```python
from build123d import *

# Parameters (mm, degrees)
SKETCH1_R           = 7.9375
SKETCH1_R_2         = 4.9657
BOSS_EXTRUDE1_DEPTH = 0.8128
FILLET1_R           = 0.32512


with BuildPart() as part:
    # Sketch1 → Boss-Extrude1 (new, symmetric)
    with BuildSketch(Plane(origin=(0, 0, 0), x_dir=(0, 0, -1), z_dir=(1, 0, 0))):
        Circle(SKETCH1_R)
        Circle(SKETCH1_R_2, mode=Mode.SUBTRACT)
    extrude(amount=BOSS_EXTRUDE1_DEPTH, both=True)

    # Fillet1
    fillet1_edges = [part.edges().sort_by_distance(p)[0] for p in [
        (-0.8128, 0, 7.9375),
        (0.8128, 0, 7.9375),
        (-0.8128, 0, 4.9657),
        (0.8128, 0, 4.9657),
    ]]
    fillet(fillet1_edges, radius=FILLET1_R)


solid = part.part
```
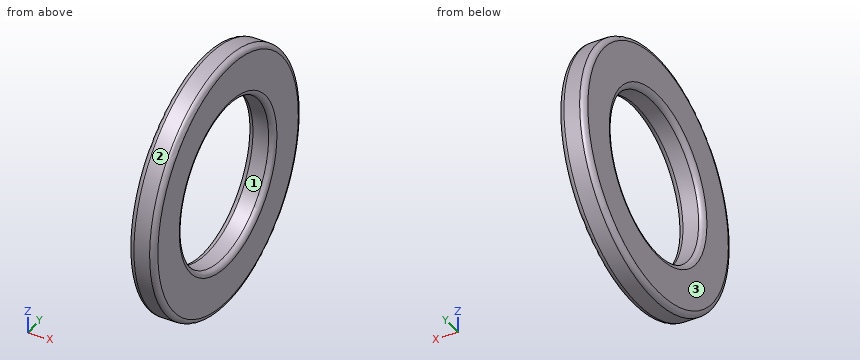
Here's how the part is built. I have some questions about the finished solid (model axes, mm). Face numbers are marked on the shaded views. Round coordinates to 2 decimals unless told otherwise and drop trailing zeros. Write each loop counter-clockwise with the first axis right and the second up, starting at its lowest first coordinate (ties: lowest second). Pieces come first, ordered by that corner, then holes.
Q1. Will this pin go through, and if not, where does the flat tip stop? P1, Ø3, axis at y = 1.5, z = 1.5, coming from the -X side.
Q2. If we section it at C-C on x = 0.1: Write out the boundary of the cut face in (y, z) (1 decimal).
Q3. If we section it at A-A on z = 0: Write out the boundary of the cut face in (x, y), plus the area to 3 significant figures.
Q4. Please list where these lines run through material, in increasing order: probe 1 along Y at (x, z) = (-0.3, 0); probe 2 along Y at (x, z) = (-0.55, -0.75); probe 3 along Z at (x, y) = (0.5, -1.75).
Q5. If we mould it in two halves opening along Z, with no side actions, what happens to the marked faces 1, 2 and 3? For each: +Z half, -Z half, draft (parallel to the pull), parting line (faces both ways), or undercut.
Answer below:
1. P1: passes through
2. outline: circle Ø15.9 at (0, 0); hole circle Ø9.9 at (0, 0)
3. outline: (-0.81, -7.61) arc R0.33 ccw to (-0.49, -7.94) - (0.49, -7.94) arc R0.33 ccw to (0.81, -7.61) - (0.81, -5.29) arc R0.33 ccw to (0.49, -4.97) - (-0.49, -4.97) arc R0.33 ccw to (-0.81, -5.29) - close; (-0.81, 5.29) arc R0.33 ccw to (-0.49, 4.97) - (0.49, 4.97) arc R0.33 ccw to (0.81, 5.29) - (0.81, 7.61) arc R0.33 ccw to (0.49, 7.94) - (-0.49, 7.94) arc R0.33 ccw to (-0.81, 7.61) - close
3. area: 9.48 mm2
4. probe 1: y = -7.94 to -4.97, 4.97 to 7.94
4. probe 2: y = -7.9 to -4.91, 4.91 to 7.9
4. probe 3: z = -7.74 to -4.65, 4.65 to 7.74
5. face 1: undercut
5. face 2: parting line
5. face 3: draft
